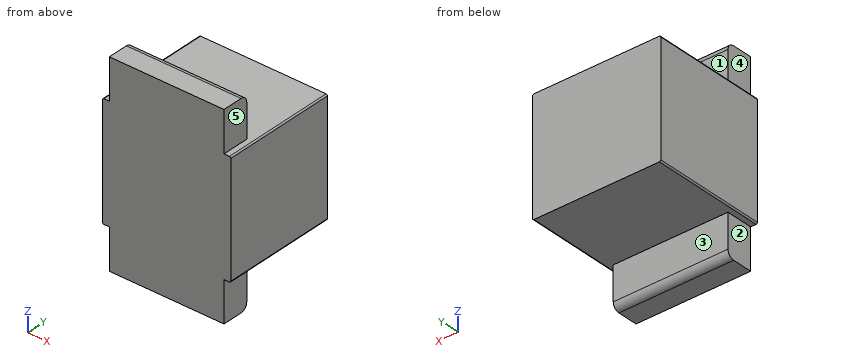
Autodesk Inventor part; units mm, degrees
ref_plane "YZ Plane" through (0, 0, 0) normal (1, 0, 0) x (0, 1, 0)
ref_plane "XZ Plane" through (0, 0, 0) normal (0, 1, 0) x (-1, 0, 0)
ref_plane "XY Plane" through (0, 0, 0) normal (0, 0, 1) x (1, 0, 0)
sketch "Sketch1" plane through (0, 0, 0) normal (0, 1, 0) x (-1, 0, 0)
  line L0 (47.5, 42.5) -> (-47.5, 42.5)
  line L1 (-47.5, 42.5) -> (-47.5, -42.5)
  line L2 (-47.5, -42.5) -> (47.5, -42.5)
  line L3 (47.5, -42.5) -> (47.5, 42.5)
  line L4 (47.5, 42.5) -> (-47.5, -42.5) construction
  line L5 (-47.5, 42.5) -> (47.5, -42.5) construction
  point P0 (0, 0)
  dimension "d0" = 95
  dimension "d1" = 85
extrude "Extrusion1" add sketch "Sketch1" along normal blind 85
fillet "Face Fillet1" radius 1 1 edges at (47.5, 42.5, 42.5)
fillet "Face Fillet2" radius 1 1 edges at (47.5, 42.5, -42.5)
fillet "Face Fillet3" radius 1 1 edges at (-47.5, 42.5, -42.5)
fillet "Face Fillet4" radius 1 1 edges at (-47.5, 42.5, 42.5)
sketch "Sketch2" plane through (46.5, 0, -42.5) normal (0, 0, -1) x (-1, 0, 0)
  line L0 (89, 0) -> (89, 20)
  line L1 (89, 20) -> (4, 20)
  line L2 (4, 20) -> (4, 0)
  line L3 (89, 0) -> (4, 0)
  point P0 (46.5, 0)
  point P1 (94, 0)
  dimension "d9" = 20
  dimension "d10" = 85
extrude "Extrusion2" add sketch "Sketch2" along normal blind 30
mirror "Mirror1" about plane through (0, 0, 0) normal (0, 0, 1) of "Extrusion2"
fillet "Face Fillet5" radius 5 1 edges at (0, 20, 72.5)
fillet "Face Fillet6" radius 5 1 edges at (0, 20, -72.5)
sketch "Sketch3" plane through (-47.5, 0, -41.5) normal (-1, 0, 0) x (0, 0, 1)
  point P0 (41.5, 0)
properties part number "base_of_linear_motor"
Geometry: final body of the model. Coordinates: model frame, mm. Face numbers are marked on the shaded views. A direction names the side the tool comes from. Round coordinates to 2 decimals unless told otherwise and drop trailing zeros. Order: outer loops, then holes, each group sorted by start corner. A loop starts at its lowest first (then second) coordinate and runs counter-clockwise, first axis right, second up. Notation, with made-up numbers: (-13, 80.5) -> (10, 80.5) arc R22 ccw to (10, 108.5) -> close; hole circle Ø9 at (3, 53.25). An arc over 180 degrees is marked (long way). Use one line per item in the form item = value. Start each with the question number.
1. Cut plane B-B (x = 10). Return the cut outline in (y, z).
2. Line query: probe 1 along Z at (x, y) = (8.5, 40.5); probe 2 along Y at (x, z) = (-17, -55); probe 3 along Z at (x, y) = (-23, 19.5). Output: solid intervals per line, ascending.
3. Cut plane A-A (y = 35.5). Return the cut outline in (x, z), then the cut area to 3 significant figures.
4. Cut plane D-D (y = 9.5). Return the cut outline in (x, z).
5. Pin query (flat end, axial travel): pin 1 Ø6 at (y, z) = (14.5, -57) entering from -X; pin 2 Ø10 at (x, y) = (-32, 68.5) entering from +Z; pin 3 Ø12 at (x, y) = (31, 30) entering from -Z. Return the tip coordinate at first contact, or that it passes through.
6. Cut plane C-C (z = 58.5). Return the cut outline in (x, y).
7. Reachability of the marked faces 1, 2, 3, 4 and 5 from +Z, -Z, +X, -X, +Y, -Y: full face, straight path, thin tool, end or side. Return the list, or none.
Solution:
q1.outline = (0, -72.5) -> (15, -72.5) arc R5 ccw to (20, -67.5) -> (20, -42.5) -> (85, -42.5) -> (85, 42.5) -> (20, 42.5) -> (20, 67.5) arc R5 ccw to (15, 72.5) -> (0, 72.5) -> close
q2.probe_1 = -42.5 to 42.5
q2.probe_2 = 0 to 20
q2.probe_3 = -69.68 to 69.68
q3.outline = (-47.5, -41.5) arc R1 ccw to (-46.5, -42.5) -> (46.5, -42.5) arc R1 ccw to (47.5, -41.5) -> (47.5, 41.5) arc R1 ccw to (46.5, 42.5) -> (-46.5, 42.5) arc R1 ccw to (-47.5, 41.5) -> close
q3.area = 8,070 mm^2
q4.outline = (-47.5, -41.5) arc R1 ccw to (-46.5, -42.5) -> (-42.5, -42.5) -> (-42.5, -72.5) -> (42.5, -72.5) -> (42.5, -42.5) -> (46.5, -42.5) arc R1 ccw to (47.5, -41.5) -> (47.5, 41.5) arc R1 ccw to (46.5, 42.5) -> (42.5, 42.5) -> (42.5, 72.5) -> (-42.5, 72.5) -> (-42.5, 42.5) -> (-46.5, 42.5) arc R1 ccw to (-47.5, 41.5) -> close
q5.pin_1 = -42.5
q5.pin_2 = 42.5
q5.pin_3 = -42.5
q6.outline = (-42.5, 0) -> (42.5, 0) -> (42.5, 20) -> (-42.5, 20) -> close
q7.face_1 = +Z, +X, -X, +Y
q7.face_2 = -Z, -X, +Y, -Y
q7.face_3 = -Z, +X, -X, +Y
q7.face_4 = +Z, -X, +Y, -Y
q7.face_5 = +Z, +X, +Y, -Y
